```python
from build123d import *

# Parameters (mm, degrees)
SKETCH2_R           = 1.331799604
BOSS_EXTRUDE1_DEPTH = 6


with BuildPart() as part:
    # Sketch2 → Boss-Extrude1 (new body)
    with BuildSketch(Plane.XY):
        with BuildLine():
            Line((-7.706246934, 57.951214685), (7.372918204, 57.951214685))
            add(Edge.make_bspline(
                [(7.372918204, 57.951214685), (7.395110156, 57.950651705), (7.438614819, 57.949548051), (7.504225261, 57.950625459), (7.555781235, 57.971549168), (7.594142025, 57.993251928), (7.6196821, 58.014176428), (7.635431909, 58.027775879), (7.643125702, 58.03441922)],
                knots=[0, 0, 0, 0, 0.227492727, 0.445972237, 0.663373124, 0.787115425, 0.896005733, 1, 1, 1, 1], degree=3))
            Line((7.643125702, 58.03441922), (10.59644992, 60.987402087))
            add(Edge.make_bspline(
                [(10.59644992, 60.987402087), (10.625456983, 61.026663762), (10.683538077, 61.105277754), (10.707695299, 61.253447318), (10.680583073, 61.389397251), (10.630907962, 61.470381818), (10.600692174, 61.504449729), (10.59644991, 61.50900292)],
                knots=[0, 0, 0, 0, 0.104345134, 0.208931166, 0.313565445, 0.39799532, 0.411364921, 0.411364921, 0.411364921, 0.411364921], degree=3))
            ThreePointArc((10.59644991, 61.50900292), (13.175131131, 60.020629535), (14.637581092, 57.427158448))
            add(Edge.make_bspline(
                [(14.637581092, 57.427158448), (14.63281413, 57.431646623), (14.598617329, 57.462223659), (14.517454165, 57.512357762), (14.3814295, 57.53955279), (14.232961651, 57.515207684), (14.154478031, 57.456521872), (14.115208769, 57.42715844)],
                knots=[0.58753787, 0.58753787, 0.58753787, 0.58753787, 0.601601228, 0.686034701, 0.790672378, 0.895262972, 1, 1, 1, 1], degree=3))
            Line((14.115208769, 57.42715844), (11.198386433, 54.510673236))
            add(Edge.make_bspline(
                [(11.198386433, 54.510673236), (11.189737643, 54.50058532), (11.172712209, 54.480726918), (11.146988546, 54.45027591), (11.11992052, 54.414228702), (11.108014065, 54.36337785), (11.109113984, 54.30464265), (11.112305892, 54.263909284), (11.114003119, 54.242250215)],
                knots=[0, 0, 0, 0, 0.134581529, 0.264928249, 0.404990742, 0.58604785, 0.779890073, 1, 1, 1, 1], degree=3))
            Line((11.114003119, 54.242250215), (11.114003119, 39.164130765))
            add(Edge.make_bspline(
                [(11.114003119, 39.164130765), (11.026069958, 38.560039142), (10.85421565, 37.379418015), (9.491383713, 36.016723245), (8.31051879, 35.844259059), (7.706108935, 35.755985581)],
                knots=[0, 0, 0, 0, 0.33840601, 0.661371999, 1, 1, 1, 1], degree=3))
            Line((7.706108935, 35.755985581), (-7.3716965, 35.755985581))
            add(Edge.make_bspline(
                [(-7.3716965, 35.755985581), (-7.390791848, 35.757243364), (-7.42588813, 35.759555105), (-7.480435634, 35.756767712), (-7.526608025, 35.741130321), (-7.568839822, 35.721664455), (-7.605836087, 35.699368029), (-7.62980257, 35.681485074), (-7.642317826, 35.672146626)],
                knots=[0, 0, 0, 0, 0.196745559, 0.361608386, 0.557261599, 0.692766378, 0.839563136, 1, 1, 1, 1], degree=3))
            Line((-7.642317826, 35.672146626), (-10.595729808, 32.719076005))
            add(Edge.make_bspline(
                [(-10.595729808, 32.719076005), (-10.624701104, 32.679767795), (-10.682693852, 32.601083323), (-10.706716869, 32.452917901), (-10.679538616, 32.31693156), (-10.627669532, 32.232998542), (-10.594437458, 32.196738778), (-10.58754182, 32.189777291)],
                knots=[0, 0, 0, 0, 0.104384754, 0.208950226, 0.313569176, 0.398093487, 0.419151196, 0.419151196, 0.419151196, 0.419151196], degree=3))
            Line((-10.58754182, 32.189777291), (-14.637683818, 36.278595616))
            add(Edge.make_bspline(
                [(-14.637683818, 36.278595616), (-14.633122591, 36.274312936), (-14.5989743, 36.243764471), (-14.518175826, 36.193440108), (-14.381934797, 36.166179863), (-14.233405716, 36.190514922), (-14.154618978, 36.249229011), (-14.11521277, 36.278595623)],
                knots=[0.587566394, 0.587566394, 0.587566394, 0.587566394, 0.601007159, 0.685956809, 0.790142009, 0.895036806, 1, 1, 1, 1], degree=3))
            Line((-14.11521277, 36.278595623), (-11.198029632, 39.195441586))
            add(Edge.make_bspline(
                [(-11.198029632, 39.195441586), (-11.190093681, 39.205582441), (-11.174520458, 39.225482487), (-11.15027016, 39.255165521), (-11.125422855, 39.293499099), (-11.110689079, 39.344394677), (-11.107300881, 39.404327233), (-11.111709764, 39.443939019), (-11.114003119, 39.464543755)],
                knots=[0, 0, 0, 0, 0.131285455, 0.257629811, 0.390972346, 0.594165008, 0.788898108, 1, 1, 1, 1], degree=3))
            Line((-11.114003119, 39.464543755), (-11.114003119, 54.542930501))
            add(Edge.make_bspline(
                [(-11.114003119, 54.542930501), (-11.025772384, 55.146864843), (-10.853333144, 56.327201592), (-9.491346414, 57.690256382), (-8.310575854, 57.862869665), (-7.706246934, 57.951214685)],
                knots=[0, 0, 0, 0, 0.338409749, 0.6613922, 1, 1, 1, 1], degree=3))
        make_face()
        with Locations((10.890728729, 57.759012308)):
            Circle(SKETCH2_R, mode=Mode.SUBTRACT)
        with BuildLine():
            Line((-0.443808512, 55.984274583), (-5.297244805, 51.131120289))
            ThreePointArc((-5.297244805, 51.131120289), (0, 37.672973009), (5.297244805, 51.131120289))
            Line((5.297244805, 51.131120289), (0.407829784, 55.984274583))
            add(Edge.make_bspline(
                [(0.407829784, 55.984274583), (0.368694639, 56.018150383), (0.291347372, 56.085103007), (0.15161935, 56.154367662), (0.050542727, 56.164189345), (5.56e-05, 56.169095213)],
                knots=[0, 0, 0, 0, 0.338885039, 0.6697773, 1, 1, 1, 1], degree=3))
            add(Edge.make_bspline(
                [(5.56e-05, 56.169095213), (-0.05257804, 56.164008855), (-0.160972548, 56.153533933), (-0.315204963, 56.089735455), (-0.401165502, 56.019243828), (-0.443808512, 55.984274583)],
                knots=[0, 0, 0, 0, 0.322338023, 0.663827768, 1, 1, 1, 1], degree=3))
        make_face(mode=Mode.SUBTRACT)
    extrude(amount=BOSS_EXTRUDE1_DEPTH)


solid = part.part
```
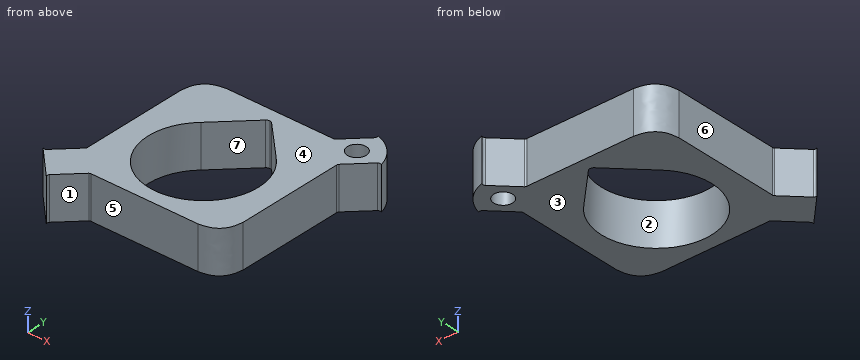
For this review, take the finished solid that the model builds, in its own axes (mm). Face numbers are marked on the shaded views. A direction names the side the tool comes from. Round coordinates to 2 decimals unless told otherwise and drop trailing zeros. Write each loop counter-clockwise with the first axis right and the second up, starting at its lowest first coordinate (ties: lowest second). Pieces come first, ordered by that corner, then holes. Notation, with made-up numbers: (88.25, 65) - (125.25, 65) arc R8 ccw to (125.25, 76) - close; hole circle Ø2 at (-32, 5.5). An arc over 180 degrees is marked (long way). Answer as a JSON object with one key per item and string values.
1. We need section A-A on y = 52.5. Give the boundary of the cut face in (x, z), then the cut area to 3 significant figures.
Response values:
{"outline": "(-11.11, 0) - (-3.93, 0) - (-3.93, 6) - (-11.11, 6) - close; (3.92, 0) - (11.11, 0) - (11.11, 6) - (3.92, 6) - close", "area": "86.3 mm2"}
2. To check wall thickness, follow line 1 along X through (y, z) = (44.5, 4); line 2 along Y through (x, z) = (0, 2.75); line 3 along Y through (x, z) = (-6, 2). State the ranges of each line that lie inside material, in increasing order.
Response values:
{"line 1": "x = -11.11 to -7.71, 7.71 to 11.11", "line 2": "y = 35.76 to 37.67, 56.17 to 57.95", "line 3": "y = 35.76 to 40.51, 50.38 to 57.95"}
3. We need section C-C on z = 2. Count the separate pieces of the cut face and the enclosed holes in it, then the cut area to 3 significant figures.
Response values:
{"separate pieces": "1", "enclosed holes": "2", "area": "317 mm2"}
4. Draft analysis for pull direction Y (two halves, no side actions). For the marked faces 1, 2 and 3, state which applies: +Y half, -Y half, draft (parallel to the pull), parting line (faces both ways), or undercut.
Response values:
{"face 1": "-Y half", "face 2": "undercut", "face 3": "draft"}
5. Tool access review of the marked faces 4, 5, 6 and 7: name each direction out of +Z, -Z, +X, -X, +Y, -Y from which nothing blocks a thin tool from reaching the whole face with its end or side.
Response values:
{"face 4": "+Z, +X, -X, +Y, -Y", "face 5": "+Z, -Z, +X, -Y", "face 6": "+Z, -Z, -X, +Y", "face 7": "+Z, -Z"}
6. For pin 1 Ø1.5 at (x, y) = (-3.5, 39) entering from +Z; pin 2 Ø1.8 at (y, z) = (46, 2) entering from -X; pin 3 Ø3 at (y, z) = (46.5, 2) entering from +X; pin 4 Ø3 at (x, z) = (3.5, 4.5) entering from -Y, all flat-tipped, find the tip position at first contact; note any pin that passes through.
Response values:
{"pin 1": "stops at z = 6", "pin 2": "stops at x = -11.11", "pin 3": "stops at x = 11.11", "pin 4": "stops at y = 35.76"}
7. We need section B-B on y = 42.5. Give the boundary of the cut face in (x, z), then the cut area to 3 significant figures.
Response values:
{"outline": "(-11.11, 0) - (-7.19, 0) - (-7.19, 6) - (-11.11, 6) - close; (7.19, 0) - (11.11, 0) - (11.11, 6) - (7.19, 6) - close", "area": "47.1 mm2"}
